```python
from build123d import *

# Parameters (mm, degrees)
SKETCH1_R           = 9
BOSS_EXTRUDE1_DEPTH = 2
FILLET1_R           = 0.5
SKETCH11_R          = 0.9
BOSS_EXTRUDE5_DEPTH = 0.3
SKETCH14_R          = 1
CUT_EXTRUDE1_DEPTH  = 40.252373603


with BuildPart() as part:
    # Sketch1 → Boss-Extrude1 (new body)
    with BuildSketch(Plane(origin=(0, 0, 0), x_dir=(1, 0, 0), z_dir=(0, 1, 0))):
        Circle(SKETCH1_R)
    extrude(amount=BOSS_EXTRUDE1_DEPTH)

    # Fillet1
    fillet1_edges = [part.edges().sort_by_distance(p)[0] for p in [
        (-9, 0, 0),
        (-9, 2, 0),
    ]]
    fillet(fillet1_edges, radius=FILLET1_R)

    # Sketch11 → Boss-Extrude5 (add)
    with BuildSketch(Plane.XY.offset(5)):
        with BuildLine():
            Line((6.549863489, 1.669069214), (11.12076654, 36.105315389))
            ThreePointArc((11.12076654, 36.105315389), (7.973708326, 39.252373603), (4.826650112, 36.105315389))
            Line((4.826650112, 36.105315389), (-6.731624766, 1.669069214))
            Line((-6.731624766, 1.669069214), (6.549863489, 1.669069214))
        make_face()
        with Locations((8.238882634, 36.669069214)):
            Circle(SKETCH11_R, mode=Mode.SUBTRACT)
    boss_extrude5 = extrude(amount=BOSS_EXTRUDE5_DEPTH)

    # Mirror1: Boss-Extrude5 across plane
    add(boss_extrude5.mirror(Plane.XY))

    # Sketch14 → Cut-Extrude1 (cut, through all)
    with BuildSketch(Plane.XZ):
        Circle(SKETCH14_R)
    extrude(amount=-CUT_EXTRUDE1_DEPTH, mode=Mode.SUBTRACT)


solid = part.part
```
Here's how the part is built. I have some questions about the finished solid (model axes, mm). A direction names the side the tool comes from. Coordinates: 2 decimals unless noted, no trailing zeros. Order: outer loops, then holes, each group sorted by start corner. A loop starts at its lowest first (then second) coordinate and runs counter-clockwise, first axis right, second up. Notation, with made-up numbers: (70.5, 49) - (112.5, 49) arc R33 ccw to (112.5, 79) - close; hole circle Ø7 at (-11, 83). An arc over 180 degrees is marked (long way). One line per question, with ' | ' between items. Start each with the question number.
1. If we section it at D-D (y = 34.5): Write out the boundary of the cut face in (x, z).
2. If we section it at A-A (z = 0): Write out the boundary of the cut face in (x, y).
3. If we section it at B-B (y = 17): Write out the boundary of the cut face in (x, z).
4. If we section it at C-C (x = 0): Write out the boundary of the cut face in (y, z) (3 decimals).
5. Which directions (+Z, -Z, +X, -X, +Y, -Y) give clear straight access to the entire face, cutting with the end or side of a thin tool? Please do faces 1 (the flat face through (4, 17, -5)), 2 (the cylindrical face through (8.65, 35.87, -5.15)), 3 (the flat face through (4, 17, -5.3)).
6. Please list where these lines run through material, in increasing order: line 1 along Z through (x, y) = (3.5, 12); line 2 along Z through (x, y) = (0, 1.3); line 3 along Y through (x, z) = (-7, 2.5). Write a range as [from, to].
7. If we mould it in two halves opening along X, with no side actions, what happens to faces 4 (the cylindrical face through (0, 1, -1)), 5 (the cylindrical face through (8.65, 35.87, 5.15)), 6 (the flat face through (4, 17, 5.3)), 7 (the cylindrical face through (-1.172, 0.993, -8.923))? For each: released by +X, released by -X, zero draft, split by the parting line, or undercut.
8. I'm going to push flat-ended pins straight in: pin 1 Ø1.6 at (x, z) = (0, 0) entering from +Y; pin 2 Ø2 at (x, z) = (-4, -1) entering from +Y; pin 3 Ø8 at (y, z) = (21, -2) entering from -X; pin 4 Ø6 at (x, y) = (7.5, 33.5) entering from +Z. Where does each tip first touch, or does it pass through?
Model answer:
1) outline: (4.29, -5.3) - (10.91, -5.3) - (10.91, -5) - (4.29, -5) - close; (4.29, 5) - (10.91, 5) - (10.91, 5.3) - (4.29, 5.3) - close
2) outline: (-9, 0.5) arc R0.5 ccw to (-8.5, 0) - (-1, 0) - (-1, 2) - (-8.5, 2) arc R0.5 ccw to (-9, 1.5) - close; (1, 0) - (8.5, 0) arc R0.5 ccw to (9, 0.5) - (9, 1.5) arc R0.5 ccw to (8.5, 2) - (1, 2) - close
3) outline: (-1.59, -5.3) - (8.58, -5.3) - (8.58, -5) - (-1.59, -5) - close; (-1.59, 5) - (8.58, 5) - (8.58, 5.3) - (-1.59, 5.3) - close
4) outline: (0, -8.5) arc R0.5 ccw to (0.5, -9) - (1.5, -9) arc R0.5 ccw to (2, -8.5) - (2, -5.3) - (21.725, -5.3) - (21.725, -5) - (2, -5) - (2, -1) - (0, -1) - close; (0, 1) - (2, 1) - (2, 5) - (21.725, 5) - (21.725, 5.3) - (2, 5.3) - (2, 8.5) arc R0.5 ccw to (1.5, 9) - (0.5, 9) arc R0.5 ccw to (0, 8.5) - close
5) face 1: +X, -X, +Y | face 2: +Z, -Z | face 3: -Z, +X, -X, +Y
6) line 1: z = [-5.3, -5], [5, 5.3] | line 2: z = [-9, -1], [1, 9] | line 3: y = [0, 2]
7) face 4: undercut | face 5: undercut | face 6: zero draft | face 7: split by the parting line
8) pin 1: passes through | pin 2: stops at y = 2 | pin 3: stops at x = -1.13 | pin 4: stops at z = 5.3
